The model under review builds one solid part; all positions refer to its coordinate system, in mm. Round coordinates to 2 decimals unless told otherwise and drop trailing zeros. Order: outer loops, then holes, each group sorted by start corner. A loop starts at its lowest first (then second) coordinate and runs counter-clockwise, first axis right, second up.
```python
from build123d import *

# Parameters (mm, degrees)
F0_R     = 95.25
F0_R_2   = 38.1
F1_DEPTH = 25.4
F2_D     = 19.84248


with BuildPart() as f1:
    # F0 (on Front) → F1 (new body)
    with BuildSketch(Plane.XZ):
        Circle(F0_R)
        Circle(F0_R_2, mode=Mode.SUBTRACT)
    extrude(amount=F1_DEPTH)

    # F2 (through all)
    with Locations(Plane(origin=(0, 0, 0), x_dir=(1, 0, 0), z_dir=(0, 1, 0))):
        with Locations((-76.2, 0), (0, -76.2), (76.2, 0), (0, 76.2)):
            Hole(F2_D / 2)


solid = f1.part
```
(1) To check wall thickness, follow probe 1 along Z at (x, y) = (0, -11.75); probe 2 along Z at (x, y) = (-5.5, -18.25); probe 3 along X at (y, z) = (-20.5, 7). State the ranges of each line that lie inside material, in increasing order.
Data:
probe 1: z = -95.25 to -86.12, -66.28 to -38.1, 38.1 to 66.28, 86.12 to 95.25
probe 2: z = -95.09 to -84.46, -67.94 to -37.7, 37.7 to 67.94, 84.46 to 95.09
probe 3: x = -94.99 to -83.23, -69.17 to -37.45, 37.45 to 69.17, 83.23 to 94.99
(2) Consider section B-B (z = -76.2). Write out the cut boundary in (x, y).
Data:
outline: (-57.15, -25.4) - (-9.92, -25.4) - (-9.92, 0) - (-57.15, 0) - close; (9.92, -25.4) - (57.15, -25.4) - (57.15, 0) - (9.92, 0) - close
(3) Consider section A-A (x = -76.2). Write out the cut boundary in (y, z), and give its area (3 significant figures).
Data:
outline: (-25.4, -57.15) - (0, -57.15) - (0, -9.92) - (-25.4, -9.92) - close; (-25.4, 9.92) - (0, 9.92) - (0, 57.15) - (-25.4, 57.15) - close
area: 2,400 mm2
(4) Consider section D-D (y = -18.25). Write out the cut boundary in (x, z).
Data:
outline: circle Ø190.5 at (0, 0); hole circle Ø19.84 at (-76.2, 0); hole circle Ø76.2 at (0, 0); hole circle Ø19.84 at (0, -76.2); hole circle Ø19.84 at (0, 76.2); hole circle Ø19.84 at (76.2, 0)
(5) Consider section C-C (z = 0). Write out the cut boundary in (x, y).
Data:
outline: (-95.25, -25.4) - (-86.12, -25.4) - (-86.12, 0) - (-95.25, 0) - close; (-66.28, -25.4) - (-38.1, -25.4) - (-38.1, 0) - (-66.28, 0) - close; (38.1, -25.4) - (66.28, -25.4) - (66.28, 0) - (38.1, 0) - close; (86.12, -25.4) - (95.25, -25.4) - (95.25, 0) - (86.12, 0) - close
(6) Draft analysis for pull direction Z (two halves, no side actions). For faces 1 (the cylindrical face through (-75.587, -12.522, -57.958)), 2 (the flat face through (-1, -25.4, -41)), 3 (the cylindrical face through (66.737, -12.878, -2.98)), state which applies: pulls with the +Z half, pulls with the -Z half, needs draft (parallel to the pull), parting line crosses it, or undercut.
Data:
face 1: parting line crosses it
face 2: needs draft
face 3: undercut
(7) Insertion check: pin 1 (6 mm diameter, centred on x = -56.5, y = -6, fed in from +Z); pin 2 (1.5 mm diameter, centred on x = -55.5, y = -19, fed in from -Z); pin 3 (4 mm diameter, centred on y = -3, z = -15, fed in from -X). Each pin has a flat end and moves straight along its axis. Give the tip position at first contact, or say it passes through.
Data:
pin 1: stops at z = 78.81
pin 2: stops at z = -77.94
pin 3: stops at x = -94.36
